from build123d import *

# Parameters (mm, degrees)
F0_R      = 20
F2_DEPTH  = 20
F4_DEPTH  = 20.001
F6_DEPTH  = 20.001
F8_W      = 40
F8_H      = 15
F12_SIZE  = 1
F7_R      = 5
F13_DEPTH = 60.001
F10_R     = 1


with BuildPart() as f2:
    # F0 (on Front) → F2 (new body)
    with BuildSketch(Plane.XZ):
        Circle(F0_R)
    extrude(amount=F2_DEPTH)

    # F3 (on face) → F4 (cut, through all)
    with BuildSketch(Plane.XZ.offset(20)):
        with BuildLine():
            Line((-18, -8.717798), (-18, 8.717798))
            ThreePointArc((-18, 8.717798), (-20, 0), (-18, -8.717798))
        make_face()
    extrude(amount=-F4_DEPTH, mode=Mode.SUBTRACT)

    # F5 (on face) → F6 (cut, through all)
    with BuildSketch(Plane.XZ.offset(20)):
        with BuildLine():
            ThreePointArc((18, -8.717798), (20, 0), (18, 8.717798))
            Line((18, 8.717798), (18, -8.717798))
        make_face()
    extrude(amount=-F6_DEPTH, mode=Mode.SUBTRACT)

    # F8 (on Right) → F11 (revolve)
    with BuildSketch(Plane.YZ):
        with Locations((20, 7.5)):
            Rectangle(F8_W, F8_H)
    revolve(axis=Axis((0, 20, 0), (0, 1, 0)))

    # F12
    f12_edges = [f2.edges().sort_by_distance(p)[0] for p in [
        (0, 40, -15),
    ]]
    chamfer(f12_edges, length=F12_SIZE)

    # F7 (on face) → F13 (cut, through all)
    with BuildSketch(Plane.XZ.offset(20)):
        Circle(F7_R)
    extrude(amount=-F13_DEPTH, mode=Mode.SUBTRACT)

    # F10 (on face) → F14 (revolve, cut)
    with BuildSketch(Plane.YZ):
        with Locations((30, 14.820702)):
            Circle(F10_R)
    revolve(axis=Axis((0, 4.966939, 0), (0, 1, 0)), mode=Mode.SUBTRACT)


solid = f2.part
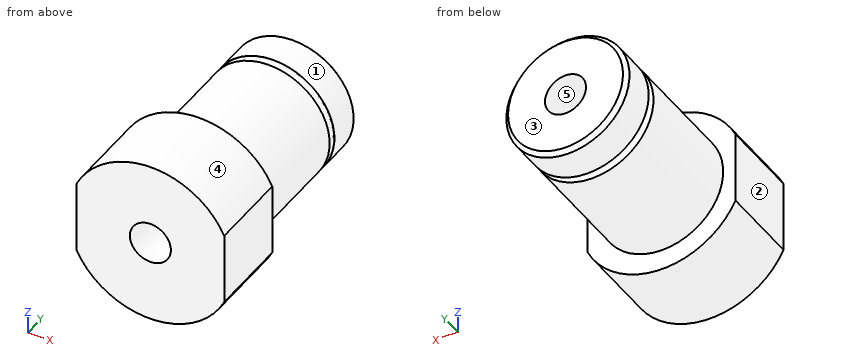
For this review, take the finished solid that the model builds, in its own axes (mm). Face numbers are marked on the shaded views. A direction names the side the tool comes from. Give positions to 0.01 mm unless a question says otherwise; leave off trailing zeros. Order: outer loops, then holes, each group sorted by start corner. A loop starts at its lowest first (then second) coordinate and runs counter-clockwise, first axis right, second up. Notation, with made-up numbers: (70, 30) - (117, 30) arc R17 ccw to (117, 38) - close; hole circle Ø2 at (16.5, 59). An arc over 180 degrees is marked (long way). Answer as a JSON object with one key per item and string values. Group by question number.
Item 1: Take a section at C-C on y = -13.5. Give the boundary of the cut face in (x, z).
Item 2: Machinability: for the marked faces 1 and 2, which of the approach directions +Z, -Z, +X, -X, +Y, -Y give a long, thin tool a straight path to every point of the face, cutting with its end or side? Answer none if there is none.
Item 3: Take a section at B-B on z = 0. Give the boundary of the cut face in (x, y), and give its area (3 significant figures).
Item 4: Take a section at A-A on x = 0. Give the boundary of the cut face in (y, z), and give its area (3 significant figures).
Item 5: Draft analysis for pull direction Z (two halves, no side actions). For the marked faces 3, 4 and 5, state which applies: pulls with the +Z half, pulls with the -Z half, needs draft (parallel to the pull), parting line crosses it, or undercut.
Item 6: Wall thickness on line 1 along Y through (x, z) = (0.5, -17); line 2 along Y through (x, z) = (3, 14.5); line 3 along Y through (x, z) = (14, -3.5): over which ranges is each line inside the solid? List them lowest first.
Item 7: Clearance check with flat-ended pins moving along their axes: pin 1 Ø4 at (x, y) = (11.5, 18) entering from -Z; pin 2 Ø8 at (y, z) = (33.5, -8.5) entering from +X; pin 3 Ø1 at (x, z) = (-6, -15) entering from +Y; pin 4 Ø9 at (x, z) = (0, 0) entering from -Y. State where each tip first meets the part, or that it passes through.
Item 8: Take a section at D-D on y = 22. Give the boundary of the cut face in (x, z).
Reported:
{
 "1": {"outline": "(-18, -8.72) arc R20 ccw to (18, -8.72) - (18, 8.72) arc R20 ccw to (-18, 8.72) - close; hole circle Ø10 at (0, 0)"},
 "2": {"face 1": "+Y", "face 2": "+Z, -Z, -X, +Y, -Y"},
 "3": {"outline": "(-18, -20) - (-5, -20) - (-5, 40) - (-14, 40) - (-15, 39) - (-15, 30.98) arc R1 cw (long way) to (-15, 29.02) - (-15, 0) - (-18, 0) - close; (5, -20) - (18, -20) - (18, 0) - (15, 0) - (15, 29.02) arc R1 cw (long way) to (15, 30.98) - (15, 39) - (14, 40) - (5, 40) - close", "area": "1,320 mm^2"},
 "4": {"outline": "(-20, -20) - (0, -20) - (0, -15) - (29.02, -15) arc R1 cw (long way) to (30.98, -15) - (39, -15) - (40, -14) - (40, -5) - (-20, -5) - close; (-20, 5) - (40, 5) - (40, 14) - (39, 15) - (30.98, 15) arc R1 cw (long way) to (29.02, 15) - (0, 15) - (0, 20) - (-20, 20) - close", "area": "1,400 mm^2"},
 "5": {"face 3": "needs draft", "face 4": "pulls with the +Z half", "face 5": "undercut"},
 "6": {"line 1": "-20 to 0", "line 2": "-20 to 29, 31 to 39.19", "line 3": "-20 to 29.08, 30.92 to 39.57"},
 "7": {"pin 1": "z = -11.61", "pin 2": "x = 14.31", "pin 3": "y = 0", "pin 4": "through"},
 "8": {"outline": "circle Ø30 at (0, 0); hole circle Ø10 at (0, 0)"}
}
